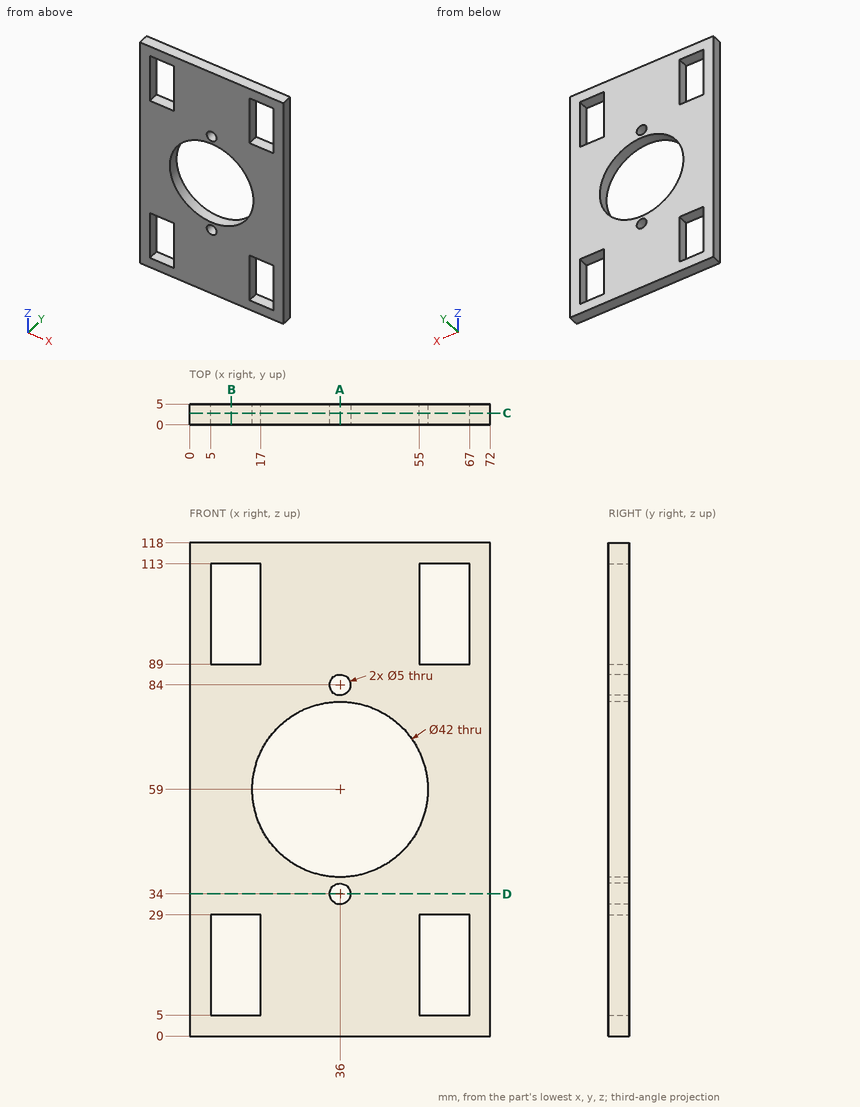
Answer from the drawing. Dimensions are ordinates in mm from the lowest x, y and z of the part. Coordinates: 2 decimals unless noted, no trailing zeros. Write each loop counter-clockwise with the first axis right and the second up, starting at its lowest first coordinate (ties: lowest second). Pieces come first, ordered by that corner, then holes. Notation, with made-up numbers: M 29.25,-1 L 83.25,-1 A23 ccw 83.25,13 Z; hole C -23,-34 d1. An arc over 180 degrees is marked long. Use a Markdown table: item, result.
Q1. The part is cut by section C-C, the plane y = 2.8. Write down the section's boundary in (x, z).
Answer block:
| item | result |
|---|---|
| outline | M 0,0 L 72,0 L 72,118 L 0,118 Z; hole M 5,5 L 17,5 L 17,29 L 5,29 Z; hole M 5,89 L 17,89 L 17,113 L 5,113 Z; hole C 36,59 d42; hole C 36,34 d5; hole C 36,84 d5; hole M 55,5 L 67,5 L 67,29 L 55,29 Z; hole M 55,89 L 67,89 L 67,113 L 55,113 Z |
Q2. Straight lines are drawn through the part: L1, parallel to Z at x = 61, y = 1; L2, parallel to Z at x = 36, y = 2.55; L3, parallel to X at y = 2.65, z = 23.5. For each, find the intervals that lie inside material, in ascending order. Write a range as [from, to].
Answer block:
| item | result |
|---|---|
| L1 | z = [0, 5], [29, 89], [113, 118] |
| L2 | z = [0, 31.5], [36.5, 38], [80, 81.5], [86.5, 118] |
| L3 | x = [0, 5], [17, 55], [67, 72] |
Q3. The part is cut by section A-A, the plane x = 36. Write down the section's boundary in (y, z).
Answer block:
| item | result |
|---|---|
| outline | M 0,0 L 5,0 L 5,31.5 L 0,31.5 Z; M 0,36.5 L 5,36.5 L 5,38 L 0,38 Z; M 0,80 L 5,80 L 5,81.5 L 0,81.5 Z; M 0,86.5 L 5,86.5 L 5,118 L 0,118 Z |
Q4. This flat-tipped pin is pushed along its axis until it touches: pin 1 Ø4.5 at (x, z) = (36, 34) entering from +Y. Where does it stop, or does it pass through?
Answer block:
| item | result |
|---|---|
| pin 1 | passes through |
Q5. The part is cut by section B-B, the plane x = 10. Write down the section's boundary in (y, z).
Answer block:
| item | result |
|---|---|
| outline | M 0,0 L 5,0 L 5,5 L 0,5 Z; M 0,29 L 5,29 L 5,89 L 0,89 Z; M 0,113 L 5,113 L 5,118 L 0,118 Z |
Q6. The part is cut by section D-D, the plane z = 34. Write down the section's boundary in (x, y).
Answer block:
| item | result |
|---|---|
| outline | M 0,0 L 33.5,0 L 33.5,5 L 0,5 Z; M 38.5,0 L 72,0 L 72,5 L 38.5,5 Z |
